Can you work these out from the model? Positions are in its coordinate system, mm. Face numbers are marked on the shaded views. Give positions to 0.01 mm unless a question says otherwise; leave off trailing zeros. Write each loop counter-clockwise with the first axis right and the second up, starting at its lowest first coordinate (ties: lowest second). Pieces come first, ordered by that corner, then holes. Notation, with made-up numbers: (0, 13) - (30, 13) arc R20 cw to (30, 23) - close; hole circle Ø7 at (-11, 59). An arc over 180 degrees is marked (long way). Return JSON: item names as keys, results as strings. Group by question number.
from build123d import *

# Parameters (mm, degrees)
SKETCH1_W           = 50.8
SKETCH1_H           = 76.2
SKETCH1_R           = 2.4892
BOSS_EXTRUDE1_DEPTH = 2.38125
FILLET1_R           = 6.35


with BuildPart() as part:
    # Sketch1 → Boss-Extrude1 (new body)
    # profile 1 of 3: a face of its own
    with BuildSketch(Plane(origin=(0, 0, 0), x_dir=(1, 0, 0), z_dir=(0, 1, 0))):
        with Locations((-99.145518613, -345.905622456)):
            Rectangle(SKETCH1_W, SKETCH1_H)
        with Locations(Location((-86.445518613, -326.855622456, 0), (0, 0, 90))):
            Circle(SKETCH1_R, mode=Mode.SUBTRACT)
        with Locations(Location((-86.445518613, -352.255622456, 0), (0, 0, 90))):
            Circle(SKETCH1_R, mode=Mode.SUBTRACT)
        with Locations(Location((-86.445518613, -377.655622456, 0), (0, 0, 90))):
            Circle(SKETCH1_R, mode=Mode.SUBTRACT)
        with Locations(Location((-99.145518613, -326.855622456, 0), (0, 0, 90))):
            Circle(SKETCH1_R, mode=Mode.SUBTRACT)
        with Locations(Location((-99.145518613, -352.255622456, 0), (0, 0, 90))):
            Circle(SKETCH1_R, mode=Mode.SUBTRACT)
        with Locations(Location((-99.145518613, -377.655622456, 0), (0, 0, 90))):
            Circle(SKETCH1_R, mode=Mode.SUBTRACT)
        with Locations(Location((-111.845518613, -377.655622456, 0), (0, 0, 90))):
            Circle(SKETCH1_R, mode=Mode.SUBTRACT)
        with Locations(Location((-111.845518613, -364.955622456, 0), (0, 0, 90))):
            Circle(SKETCH1_R, mode=Mode.SUBTRACT)
        with Locations(Location((-111.845518613, -352.255622456, 0), (0, 0, 90))):
            Circle(SKETCH1_R, mode=Mode.SUBTRACT)
        with Locations(Location((-111.845518613, -339.555622456, 0), (0, 0, 90))):
            Circle(SKETCH1_R, mode=Mode.SUBTRACT)
        with Locations(Location((-111.845518613, -326.855622456, 0), (0, 0, 90))):
            Circle(SKETCH1_R, mode=Mode.SUBTRACT)
        with Locations(Location((-111.845518613, -314.155622456, 0), (0, 0, 90))):
            Circle(SKETCH1_R, mode=Mode.SUBTRACT)
        with Locations(Location((-99.145518613, -364.955622456, 0), (0, 0, 90))):
            Circle(SKETCH1_R, mode=Mode.SUBTRACT)
        with Locations(Location((-99.145518613, -339.555622456, 0), (0, 0, 90))):
            Circle(SKETCH1_R, mode=Mode.SUBTRACT)
        with Locations(Location((-99.145518613, -314.155622456, 0), (0, 0, 90))):
            Circle(SKETCH1_R, mode=Mode.SUBTRACT)
        with Locations(Location((-86.445518613, -364.955622456, 0), (0, 0, 90))):
            Circle(SKETCH1_R, mode=Mode.SUBTRACT)
        with Locations(Location((-86.445518613, -339.555622456, 0), (0, 0, 90))):
            Circle(SKETCH1_R, mode=Mode.SUBTRACT)
        with Locations(Location((-86.445518613, -314.155622456, 0), (0, 0, 90))):
            Circle(SKETCH1_R, mode=Mode.SUBTRACT)
    # profile 2 of 3: a face of its own
    with BuildSketch(Plane(origin=(0, 0, 0), x_dir=(1, 0, 0), z_dir=(0, 1, 0))):
        Polygon((-73.745518613, -307.805622456), (-124.545518613, -307.805622456), (-124.545518613, -267.92136832), (-73.745518613, -286.411056221), align=None)
        with Locations(Location((-102.075911776, -280.451262674, 0), (0, 0, 90))):
            Circle(SKETCH1_R, mode=Mode.SUBTRACT)
        with Locations(Location((-114.01000806, -276.107606853, 0), (0, 0, 90))):
            Circle(SKETCH1_R, mode=Mode.SUBTRACT)
        with Locations(Location((-90.141815492, -284.794918494, 0), (0, 0, 90))):
            Circle(SKETCH1_R, mode=Mode.SUBTRACT)
    # profile 3 of 3: a face of its own
    with BuildSketch(Plane(origin=(0, 0, 0), x_dir=(1, 0, 0), z_dir=(0, 1, 0))):
        Polygon((-124.545518613, -267.92136832), (-73.745518613, -286.411056221), (-73.745518613, -276.87877894), (-54.317612196, -223.501044752), (-102.053997332, -206.126421471), align=None)
        with Locations(Location((-109.666352239, -264.173510569, 0), (0, 0, 90))):
            Circle(SKETCH1_R, mode=Mode.SUBTRACT)
        with Locations(Location((-105.322696419, -252.239414285, 0), (0, 0, 90))):
            Circle(SKETCH1_R, mode=Mode.SUBTRACT)
        with Locations(Location((-97.732255955, -268.51716639, 0), (0, 0, 90))):
            Circle(SKETCH1_R, mode=Mode.SUBTRACT)
        with Locations(Location((-93.388600135, -256.583070106, 0), (0, 0, 90))):
            Circle(SKETCH1_R, mode=Mode.SUBTRACT)
        with Locations(Location((-100.979040599, -240.305318001, 0), (0, 0, 90))):
            Circle(SKETCH1_R, mode=Mode.SUBTRACT)
        with Locations(Location((-96.635384779, -228.371221717, 0), (0, 0, 90))):
            Circle(SKETCH1_R, mode=Mode.SUBTRACT)
        with Locations(Location((-92.291728958, -216.437125433, 0), (0, 0, 90))):
            Circle(SKETCH1_R, mode=Mode.SUBTRACT)
        with Locations(Location((-85.798159671, -272.86082221, 0), (0, 0, 90))):
            Circle(SKETCH1_R, mode=Mode.SUBTRACT)
        with Locations(Location((-81.454503851, -260.926725926, 0), (0, 0, 90))):
            Circle(SKETCH1_R, mode=Mode.SUBTRACT)
        with Locations(Location((-89.044944315, -244.648973822, 0), (0, 0, 90))):
            Circle(SKETCH1_R, mode=Mode.SUBTRACT)
        with Locations(Location((-84.701288495, -232.714877538, 0), (0, 0, 90))):
            Circle(SKETCH1_R, mode=Mode.SUBTRACT)
        with Locations(Location((-77.110848031, -248.992629642, 0), (0, 0, 90))):
            Circle(SKETCH1_R, mode=Mode.SUBTRACT)
        with Locations(Location((-72.767192211, -237.058533358, 0), (0, 0, 90))):
            Circle(SKETCH1_R, mode=Mode.SUBTRACT)
        with Locations(Location((-80.357632674, -220.780781254, 0), (0, 0, 90))):
            Circle(SKETCH1_R, mode=Mode.SUBTRACT)
        with Locations(Location((-68.42353639, -225.124437074, 0), (0, 0, 90))):
            Circle(SKETCH1_R, mode=Mode.SUBTRACT)
    extrude(amount=BOSS_EXTRUDE1_DEPTH)

    # Fillet1
    fillet1_edges = [part.edges().sort_by_distance(p)[0] for p in [
        (-73.745518613, 1.190625, 384.005622456),
        (-124.545518613, 1.190625, 384.005622456),
        (-124.545518613, 1.190625, 267.92136832),
        (-102.053997332, 1.190625, 206.126421471),
        (-54.317612196, 1.190625, 223.501044752),
        (-73.745518613, 1.190625, 276.87877894),
    ]]
    fillet(fillet1_edges, radius=FILLET1_R)


solid = part.part
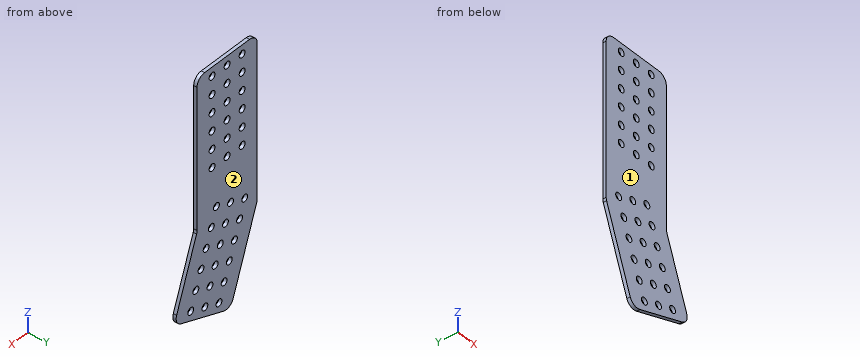
1) I need wall thicknesses on line 1 along Z through (x, y) = (-92, 0.9); line 2 along X through (y, z) = (0.65, 254.5); line 3 along X through (y, z) = (1.8, 312). Which ranges of each line are inside material? Lowest first, please.
2) Imagine slicing it at A-A, the plane z = 351.5. Write out the boundary of the cut face in (x, y), and give its area (3 significant figures).
3) Will this pin go through, and if not, where does the flat tip stop? pin 1 Ø4 at (x, z) = (-114.01, 276.11) entering from -Y.
4) Imagine slicing it at B-B, the plane z = 307.5. Write out the boundary of the cut face in (x, y).
5) Imagine slicing it at C-C, the plane y = 1. Count the separate pieces of the cut face and the enclosed holes in it, and give its area (3 significant figures).
6) We'd pull the mould along Y, two halves only. Please class the marked faces 1 and 2: pulls with the +Y half, pulls with the -Y half, needs draft (parallel to the pull), parting line crosses it, or undercut.
Resolved:
{
 "1": {"line 1": "209.79 to 213.97, 218.91 to 254.52, 258.65 to 283.14, 286.45 to 384.01", "line 2": "-119.66 to -106.36, -104.28 to -94.75, -92.03 to -65.6", "line 3": "-124.55 to -113.09, -110.6 to -100.39, -97.9 to -87.69, -85.2 to -73.75"},
 "2": {"outline": "(-124.55, 0) - (-114.22, 0) - (-114.22, 2.38) - (-124.55, 2.38) - close; (-109.47, 0) - (-101.52, 0) - (-101.52, 2.38) - (-109.47, 2.38) - close; (-96.77, 0) - (-88.82, 0) - (-88.82, 2.38) - (-96.77, 2.38) - close; (-84.07, 0) - (-73.75, 0) - (-73.75, 2.38) - (-84.07, 2.38) - close", "area": "87.1 mm^2"},
 "3": {"pin 1": "through"},
 "4": {"outline": "(-124.55, 0) - (-73.75, 0) - (-73.75, 2.38) - (-124.55, 2.38) - close"},
 "5": {"separate pieces": "1", "enclosed holes": "36", "area": "8,050 mm^2"},
 "6": {"face 1": "pulls with the -Y half", "face 2": "pulls with the +Y half"}
}
